from build123d import *

# Parameters (mm, degrees)
SKETCH_1_W          = 14
SKETCH_1_H          = 9
EXTRUDE_1_DEPTH     = 14
FILLET_1_R          = 1
SKETCH_3_R          = 1.75
CUT_EXTRUDE_2_DEPTH = 7
CUT_EXTRUDE_3_REACH = 12.874
SKETCH_4_R          = 1.05
CUT_EXTRUDE_START   = -14
SKETCH_6_W          = 0.5
SKETCH_6_H          = 9
CUT_EXTRUDE_4_DEPTH = 13


with BuildPart() as part:
    # 草图1 → 凸台-拉伸1 (new body)
    with BuildSketch(Plane(origin=(0, 0, 0), x_dir=(1, 0, 0), z_dir=(0, 1, 0))):
        Rectangle(SKETCH_1_W, SKETCH_1_H)
    extrude(amount=EXTRUDE_1_DEPTH)

    # 圆角1
    fillet_1_edges = [part.edges().sort_by_distance(p)[0] for p in [
        (7, 7, 4.5),
        (-7, 7, 4.5),
        (-7, 7, -4.5),
        (7, 7, -4.5),
    ]]
    fillet(fillet_1_edges, radius=FILLET_1_R)

    # 草图3 → 切除-拉伸2 (cut)
    with BuildSketch(Plane(origin=(0, 14, 0), x_dir=(1, 0, 0), z_dir=(0, 1, 0))):
        with Locations(Location((-2.5, 0, 0), (0, 0, 270))):
            Circle(SKETCH_3_R)
        with Locations(Location((2.5, 0, 0), (0, 0, 90))):
            Circle(SKETCH_3_R)
    extrude(amount=-CUT_EXTRUDE_2_DEPTH, mode=Mode.SUBTRACT)

    # 草图4 → 切除-拉伸3 (cut, up to next)
    with BuildSketch(Plane(origin=(0, 7, 0), x_dir=(1, 0, 0), z_dir=(0, 1, 0)), mode=Mode.PRIVATE) as cut_extrude_3_sk1:
        with Locations(Location((-2.5, 0, 0), (0, 0, 270))):
            Circle(SKETCH_4_R)
    cut_extrude_3_tool1 = extrude(cut_extrude_3_sk1.sketch, amount=-CUT_EXTRUDE_3_REACH, mode=Mode.PRIVATE) & part.part
    # 草图4 → 切除-拉伸3 (cut, up to next)
    with BuildSketch(Plane(origin=(0, 7, 0), x_dir=(1, 0, 0), z_dir=(0, 1, 0)), mode=Mode.PRIVATE) as cut_extrude_3_sk2:
        with Locations(Location((2.5, 0, 0), (0, 0, 270))):
            Circle(SKETCH_4_R)
    cut_extrude_3_tool2 = extrude(cut_extrude_3_sk2.sketch, amount=-CUT_EXTRUDE_3_REACH, mode=Mode.PRIVATE) & part.part
    add(cut_extrude_3_tool1.solids().sort_by_distance((-2.5, 7, 0))[0], mode=Mode.SUBTRACT)
    add(cut_extrude_3_tool2.solids().sort_by_distance((2.5, 7, 0))[0], mode=Mode.SUBTRACT)

    # 草图6 → 切除-拉伸4 (cut)
    with BuildSketch(Plane(origin=(0, 14, 0), x_dir=(1, 0, 0), z_dir=(0, 1, 0)).offset(CUT_EXTRUDE_START)):
        Rectangle(SKETCH_6_W, SKETCH_6_H)
    extrude(amount=CUT_EXTRUDE_4_DEPTH, mode=Mode.SUBTRACT)


solid = part.part
Input: part model. Units: mm. Frame: model coordinates. A direction names the side the tool comes from. Round coordinates to 2 decimals unless told otherwise and drop trailing zeros. Write each loop counter-clockwise with the first axis right and the second up, starting at its lowest first coordinate (ties: lowest second). Pieces come first, ordered by that corner, then holes.
1) Cut plane A-A (y = 6). Return the cut outline in (x, z), then the cut area to 3 significant figures.
2) Cut plane C-C (x = -2.5). Return the cut outline in (y, z), then the cut area to 3 significant figures.
3) Reachability of faces 1 (the flat face through (-4, 7, 0)), 2 (the cylindrical face through (-3.525, 3.549, -0.228)), 3 (the flat face through (-0.25, 6, 0)) from +Z, -Z, +X, -X, +Y, -Y: full face, straight path, thin tool, end or side. Return the list, or none.
4) Cut plane D-D (y = 8.5). Return the cut outline in (x, z).
5) Cut plane B-B (z = 0). Return the cut outline in (x, y).
6) Contact query for a flat-ended pin moving along its axis: P1, Ø1, axis at x = 3, z = -0.5, coming from the +Y side. Output: stop coordinate, or through.
7) Draft query along X for faces 4 (the cylindrical face through (4.21, 10.55, 0.38)), 5 (the flat face through (0, 14, 0)), 6 (the cylindrical face through (6.699, 7.098, 4.215)). Return one class per face: pulls with the +X half, pulls with the -X half, needs draft (parallel to the pull), parting line crosses it, or undercut.
8) Ray query, L1, parallel to X at y = 4.75, z = 0; L2, parallel to X at y = 9.25, z = 0; L3, parallel to X at y = 4, z = -2.5. Return the intervals inside material, ascending.
Geometry says:
1. outline: (-7, -3.5) arc R1 ccw to (-6, -4.5) - (-0.25, -4.5) - (-0.25, 4.5) - (-6, 4.5) arc R1 ccw to (-7, 3.5) - close; (0.25, -4.5) - (6, -4.5) arc R1 ccw to (7, -3.5) - (7, 3.5) arc R1 ccw to (6, 4.5) - (0.25, 4.5) - close; hole circle Ø2.1 at (-2.5, 0); hole circle Ø2.1 at (2.5, 0)
1. area: 114 mm2
2. outline: (0, -4.5) - (14, -4.5) - (14, -1.75) - (7, -1.75) - (7, -1.05) - (0, -1.05) - close; (0, 1.05) - (7, 1.05) - (7, 1.75) - (14, 1.75) - (14, 4.5) - (0, 4.5) - close
2. area: 86.8 mm2
3. face 1: +Y
3. face 2: +Y, -Y
3. face 3: +Z, -Z, -Y
4. outline: (-7, -3.5) arc R1 ccw to (-6, -4.5) - (-0.25, -4.5) - (-0.25, 4.5) - (-6, 4.5) arc R1 ccw to (-7, 3.5) - close; (0.25, -4.5) - (6, -4.5) arc R1 ccw to (7, -3.5) - (7, 3.5) arc R1 ccw to (6, 4.5) - (0.25, 4.5) - close; hole circle Ø3.5 at (-2.5, 0); hole circle Ø3.5 at (2.5, 0)
5. outline: (-7, 0) - (-3.55, 0) - (-3.55, 7) - (-4.25, 7) - (-4.25, 14) - (-7, 14) - close; (-1.45, 0) - (-0.25, 0) - (-0.25, 13) - (0.25, 13) - (0.25, 0) - (1.45, 0) - (1.45, 7) - (0.75, 7) - (0.75, 14) - (-0.75, 14) - (-0.75, 7) - (-1.45, 7) - close; (3.55, 0) - (7, 0) - (7, 14) - (4.25, 14) - (4.25, 7) - (3.55, 7) - close
6. P1: stops at y = 7
7. face 4: undercut
7. face 5: needs draft
7. face 6: pulls with the +X half
8. L1: x = -7 to -3.55, -1.45 to -0.25, 0.25 to 1.45, 3.55 to 7
8. L2: x = -7 to -4.25, -0.75 to -0.25, 0.25 to 0.75, 4.25 to 7
8. L3: x = -7 to -0.25, 0.25 to 7
